Here's how the part is built. I have some questions about the finished solid (model axes, mm). A direction names the side the tool comes from. Coordinates: 2 decimals unless noted, no trailing zeros. Write each loop counter-clockwise with the first axis right and the second up, starting at its lowest first coordinate (ties: lowest second). Pieces come first, ordered by that corner, then holes.
Item 1: I'm going to push flat-ended pins straight in: P1, Ø1.5, axis at y = 12.5, z = 38.5, coming from the -X side; P2, Ø0.9, axis at x = 4, z = 37.5, coming from the +Y side; P3, Ø1.6, axis at x = 3.5, y = 45, coming from the -Z side. Where does each tip first touch, or does it pass through?
Item 2: I want a section at D-D (z = 63). Please give me the cut outline in (x, y), and give its area (3 significant figures).
Item 3: For faces 1 (the face through (20.5, 105, 72)), 2 (the face through (101, 93, 53)), 3 (the face through (2, 173, 38)), 4 (the face through (52, 95, 74)), which set-ups out of +Z, -Z, +X, -X, +Y, -Y let a thin tool reach every point of the face, with its end or its side?
Item 4: I want a section at B-B (y = 79). Please give me the cut outline in (x, z).
Item 5: I want a section at C-C (x = 18). Please give me the cut outline in (y, z), and give its area (3 significant figures).
Item 6: Please list where these lines run through material, in increasing order: line 1 (X direction, y = 61, z = 60); line 2 (Y direction, x = 62, z = 43.5); line 3 (X direction, y = 37, z = 55).
Item 7: I want a section at A-A (z = 51). Please give me the cut outline in (x, y).
Item 8: If we mould it in two halves opening along Y, with no side actions, what happens to faces 5 (the face through (52, 188, 57)), 6 (the face through (52, 185, 55)), 7 (the face through (52, 0, 57))? For each: pulls with the +Y half, pulls with the -Y half, needs draft (parallel to the pull), parting line crosses it, or undercut.
from build123d import *

# Parameters (mm, degrees)
SKETCH016_W         = 106
SKETCH016_H         = 188
SKETCH016_W_2       = 96
SKETCH016_H_2       = 182
PAD010_DEPTH        = 30
SKETCH017_W         = 3
SKETCH017_H         = 15
SKETCH017_H_2       = 25
PAD011_DEPTH        = 3.8
SKETCH018_W         = 3.2
SKETCH018_H         = 21
SKETCH018_W_2       = 3.2000000001
POCKET006_DEPTH     = 16.5
SKETCH019_W         = 106
SKETCH019_H         = 188
SKETCH019_W_2       = 65
SKETCH019_H_2       = 10
PAD012_DEPTH        = 4
CHAMFER001_SIZE     = 0.8
CHAMFER002_SIZE     = 0.8
PAD013_DEPTH        = 4
LINEARPATTERN_COUNT = 35
LINEARPATTERN_PITCH = 1.7941176471


with BuildPart() as part:
    # Sketch016 → Pad010 (new body)
    with BuildSketch(Plane.XY):
        with Locations((53, 94)):
            Rectangle(SKETCH016_W, SKETCH016_H)
        with Locations((53, 94)):
            Rectangle(SKETCH016_W_2, SKETCH016_H_2, mode=Mode.SUBTRACT)
    extrude(amount=PAD010_DEPTH)

    # Sketch017 (on Face9 of Pad010) → Pad011 (join)
    with BuildSketch(Plane(origin=(0, 0, 0), x_dir=(1, 0, 0), z_dir=(0, 0, -1))):
        with Locations((3.5, -10.5)):
            Rectangle(SKETCH017_W, SKETCH017_H)
        with Locations((3.5, -172.5)):
            Rectangle(SKETCH017_W, SKETCH017_H_2)
        with Locations((102.5, -172.5)):
            Rectangle(SKETCH017_W, SKETCH017_H_2)
        with Locations((102.5, -10.5)):
            Rectangle(SKETCH017_W, SKETCH017_H)
    extrude(amount=PAD011_DEPTH)

    # Sketch018 (on Face4 of Pad011) → Pocket006 (cut)
    with BuildSketch(Plane(origin=(0, 0, 0), x_dir=(1, 0, 0), z_dir=(0, 0, -1))):
        with Locations((3.4, -45)):
            Rectangle(SKETCH018_W, SKETCH018_H)
        with Locations((102.6, -45)):
            Rectangle(SKETCH018_W_2, SKETCH018_H)
    extrude(amount=-POCKET006_DEPTH, mode=Mode.SUBTRACT)

    # Sketch019 (on Face5 of Pocket006) → Pad012 (join)
    with BuildSketch(Plane.XY.offset(30)):
        with Locations((53, 94)):
            Rectangle(SKETCH019_W, SKETCH019_H)
        with Locations((52.9999999999, 105)):
            Rectangle(SKETCH019_W_2, SKETCH019_H_2, mode=Mode.SUBTRACT)
    extrude(amount=PAD012_DEPTH)

    # Chamfer001
    chamfer001_edges = [part.edges().sort_by_distance(p)[0] for p in [
        (101, 10.5, -3.8),
        (102.5, 18, -3.8),
        (104, 10.5, -3.8),
        (102.5, 3, -3.8),
        (102.5, 185, -3.8),
        (104, 172.5, -3.8),
        (102.5, 160, -3.8),
        (101, 172.5, -3.8),
        (5, 172.5, -3.8),
        (3.5, 3, -3.8),
        (2, 10.5, -3.8),
        (3.5, 18, -3.8),
        (5, 10.5, -3.8),
    ]]
    chamfer(chamfer001_edges, length=CHAMFER001_SIZE)

    # Chamfer002
    chamfer002_edges = [part.edges().sort_by_distance(p)[0] for p in [
        (102.6, 55.5, 0),
        (102.6, 34.5, 0),
        (3.4, 34.5, 0),
        (3.4, 55.5, 0),
    ]]
    chamfer(chamfer002_edges, length=CHAMFER002_SIZE)

    # Sketch020 (on Face12 of Chamfer002) → Pad013 (join)
    with BuildSketch(Plane(origin=(0, 0, 30), x_dir=(1, 0, 0), z_dir=(0, 0, -1))):
        Polygon((84.4999999999, -100), (83.4999999999, -102), (82.4999999999, -100), align=None)
    pad013 = extrude(amount=-PAD013_DEPTH)

    # LinearPattern: Pad013 ×35
    with Locations(*[(-i * LINEARPATTERN_PITCH, 0, 0) for i in range(1, LINEARPATTERN_COUNT)]):
        add(pad013)


with BuildPart() as part_1:
    # Body003 placement: moved
    add(part.part.moved(Location((0, 0, 40))))


solid = part_1.part
Answer:
1. P1: stops at x = 2
1. P2: stops at y = 185
1. P3: stops at z = 56.5
2. outline: (0, 0) - (106, 0) - (106, 188) - (0, 188) - close; hole (5, 3) - (101, 3) - (101, 185) - (5, 185) - close
2. area: 2,460 mm2
3. face 1: +Z, -Z
3. face 2: -Z
3. face 3: -Z, -X, +Y, -Y
3. face 4: +Z, +X, -X, +Y, -Y
4. outline: (0, 40) - (5, 40) - (5, 70) - (101, 70) - (101, 40) - (106, 40) - (106, 74) - (0, 74) - close
5. outline: (0, 40) - (3, 40) - (3, 70) - (185, 70) - (185, 40) - (188, 40) - (188, 74) - (0, 74) - close
5. area: 932 mm2
6. line 1: x = 0 to 5, 101 to 106
6. line 2: y = 0 to 3, 185 to 188
6. line 3: x = 0 to 1.8, 104.2 to 106
7. outline: (0, 0) - (106, 0) - (106, 188) - (0, 188) - close; hole (1.8, 34.5) - (5, 34.5) - (5, 3) - (101, 3) - (101, 34.5) - (104.2, 34.5) - (104.2, 55.5) - (101, 55.5) - (101, 185) - (5, 185) - (5, 55.5) - (1.8, 55.5) - close
8. face 5: pulls with the +Y half
8. face 6: undercut
8. face 7: pulls with the -Y half
